Here's the drawing with two shaded views (mm, measured from the low corner). I have some questions. Round coordinates to 2 decimals unless told otherwise and drop trailing zeros. Write each loop counter-clockwise with the first axis right and the second up, starting at its lowest first coordinate (ties: lowest second). Pieces come first, ordered by that corner, then holes. Notation, with made-up numbers: M -8,57.5 L 14,57.5 A24 cw 14,83.5 Z; hole C -5,-23 d2. An arc over 180 degrees is marked long. Use one line per item in the form item = value. Start each with the question number.
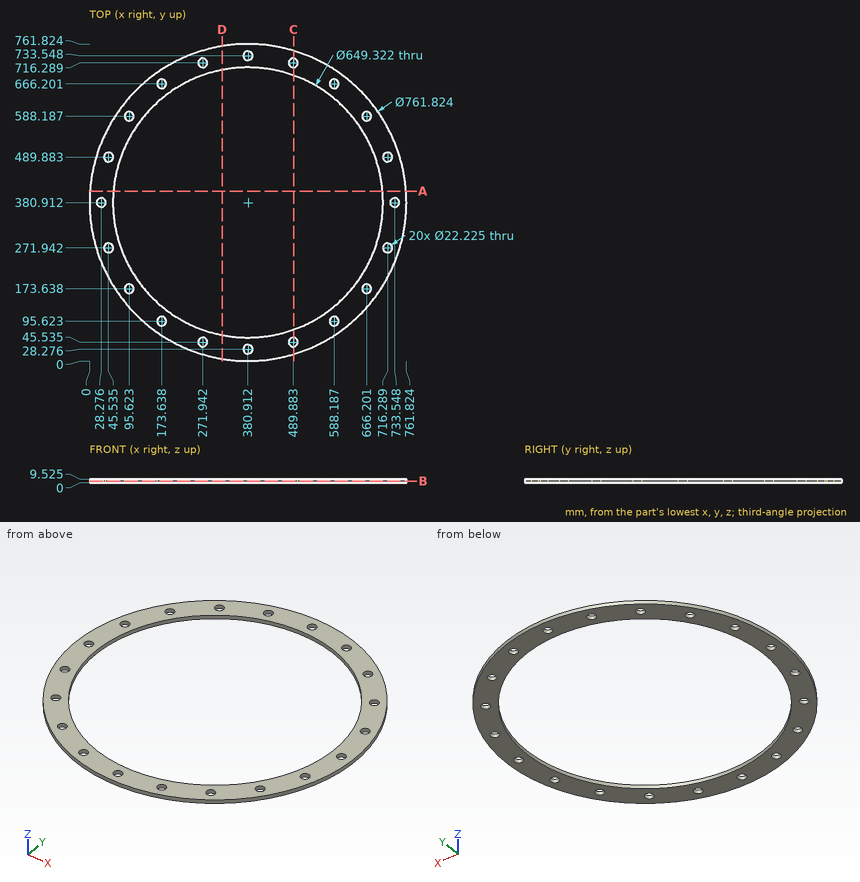
1. Will these pins go through, and if not, where does the flat tip stop? pin 1 (4 mm diameter, centred on y = 417.5, z = 1.5, fed in from -X); pin 2 (1.5 mm diameter, centred on x = 494, z = 3, fed in from -Y); pin 3 (1.5 mm diameter, centred on y = 138, z = 7, fed in from -X) (1 decimal).
2. If we section it at D-D (x = 319): List the corners of the cut face in (y, z) for me (1 decimal), and give its area (3 significant figures).
3. Please list where these lines run through material, in increasing order: line 1 along Y through (x, z) = (173, 4.75) (1 decimal); line 2 along Y through (x, z) = (271, 4.75) (1 decimal); line 3 along Y through (x, z) = (50, 9.25) (1 decimal).
4. If we section it at C-C (x = 490.5): List the corners of the cut face in (y, z) for me (1 decimal), and give its area (3 significant figures).
5. If we section it at B-B (z = 4.5): State how many separate pieces and enclosed holes the cut face has, and give its area (3 significant figures).
6. If we section it at A-A (y = 408): List the corners of the cut face in (x, z) for me (1 decimal).
Model answer:
q1.pin_1 = 1.57
q1.pin_2 = 16.94
q1.pin_3 = 86.9
q2.outline = M 5.1,0 L 62.2,0 L 62.2,9.5 L 5.1,9.5 Z; M 699.6,0 L 756.8,0 L 756.8,9.5 L 699.6,9.5 Z
q2.area = 1,090 mm2
q3.line_1 = 61.7 to 84.5, 106.7 to 131.6, 630.3 to 655.1, 677.3 to 700.1
q3.line_2 = 16.2 to 34.5, 56.6 to 75.4, 686.4 to 705.2, 727.4 to 745.6
q3.line_3 = 192.3 to 261.8, 282.1 to 479.7, 500.1 to 569.6
q4.outline = M 16.1,0 L 34.4,0 L 34.4,9.5 L 16.1,9.5 Z; M 56.6,0 L 75.3,0 L 75.3,9.5 L 56.6,9.5 Z; M 686.5,0 L 705.2,0 L 705.2,9.5 L 686.5,9.5 Z; M 727.4,0 L 745.7,0 L 745.7,9.5 L 727.4,9.5 Z
q4.area = 705 mm2
q5.separate_pieces = 1
q5.enclosed_holes = 21
q5.area = 117,000 mm2
q6.outline = M 1,0 L 57.4,0 L 57.4,9.5 L 1,9.5 Z; M 704.4,0 L 760.9,0 L 760.9,9.5 L 704.4,9.5 Z
